```python
from build123d import *

# Parameters (mm, degrees)
SM_BASE_FLANGE_1_DEPTH  = 419.5
CUT_EXTRUDE_1_DEPTH     = 492.235686814
FILLET_1_R              = 10
HOLE_WIZARD_M12_1_D     = 10.2
HOLE_WIZARD_M12_1_DEPTH = 32.75
HOLE_WIZARD_M12_1_TIP   = 3.064389157


# Sheet-metal steps are written as plain solids
with BuildPart() as part:
    # Sketch 1 → 基体-法兰1 (new, symmetric)
    with BuildSketch(Plane(origin=(0, 0, 0), x_dir=(0, 0, -1), z_dir=(1, 0, 0))):
        with BuildLine():
            Line((-115, -111.5), (-115, -20))
            ThreePointArc((-115, -20), (-109.142135624, -5.857864376), (-95, 0))
            Line((-95, 0), (95, 0))
            ThreePointArc((95, 0), (109.142135624, -5.857864376), (115, -20))
            Line((115, -20), (115, -111.5))
            Line((115, -111.5), (105, -111.5))
            Line((105, -111.5), (105, -20))
            ThreePointArc((105, -20), (102.071067812, -12.928932188), (95, -10))
            Line((95, -10), (-95, -10))
            ThreePointArc((-95, -10), (-102.071067812, -12.928932188), (-105, -20))
            Line((-105, -20), (-105, -111.5))
            Line((-105, -111.5), (-115, -111.5))
        make_face()
    extrude(amount=SM_BASE_FLANGE_1_DEPTH, both=True)

    # Sketch 2 → 切除-拉伸1 (cut, through all)
    with BuildSketch(Plane(origin=(0, 0, -115), x_dir=(-1, 0, 0), z_dir=(0, 0, -1))):
        Polygon((-214.641016151, -111.5), (-180, -51.5), (180, -51.5), (214.641016151, -111.5), align=None)
    extrude(amount=-CUT_EXTRUDE_1_DEPTH, mode=Mode.SUBTRACT)

    # 圆角1
    fillet_1_edges = [part.edges().sort_by_distance(p)[0] for p in [
        (-214.641016151, -111.5, -110),
        (214.641016151, -111.5, -110),
        (180, -51.5, -110),
        (-180, -51.5, -110),
        (214.641016151, -111.5, 110),
        (-214.641016151, -111.5, 110),
        (-180, -51.5, 110),
        (180, -51.5, 110),
    ]]
    fillet(fillet_1_edges, radius=FILLET_1_R)

    # M12 螺纹孔1
    with Locations(Plane(origin=(0, 0, 0), x_dir=(1, 0, 0), z_dir=(0, 1, 0))):
        with Locations((-110, 50), (110, 50), (110, -50), (-110, -50)):
            Hole(HOLE_WIZARD_M12_1_D / 2, depth=HOLE_WIZARD_M12_1_DEPTH)
            with Locations((0, 0, -(HOLE_WIZARD_M12_1_DEPTH + HOLE_WIZARD_M12_1_TIP / 2))):  # 118° drill point
                Cone(0, HOLE_WIZARD_M12_1_D / 2, HOLE_WIZARD_M12_1_TIP, mode=Mode.SUBTRACT)


solid = part.part
```
Build history of the part. All positions in model axes, mm. A direction names the side the tool comes from. Give positions to 0.01 mm unless a question says otherwise; leave off trailing zeros. Loops run counter-clockwise (first coordinate to the right, second up) from the corner with the lowest first, then second, coordinate; pieces in that order, holes last.
Item 1: Slice it at D-D, the plane x = 309. List the corners of the cut face in (y, z), and give its area (3 significant figures).
Answers follow:
outline: (-111.5, -115) - (-20, -115) arc R20 ccw to (0, -95) - (0, 95) arc R20 ccw to (-20, 115) - (-111.5, 115) - (-111.5, 105) - (-20, 105) arc R10 cw to (-10, 95) - (-10, -95) arc R10 cw to (-20, -105) - (-111.5, -105) - close
area: 4,200 mm2
Item 2: Flat gauge pins, fed straight in: pin 1 (1.5 mm diameter, centred on x = -240.5, y = -18.5, fed in from -Z); pin 2 (8 mm diameter, centred on x = -41.5, z = -109, fed in from -Y); pin 3 (5 mm diameter, centred on x = -168, z = 12, fed in from -Y). Where does each tip first touch, or does it go through?
Answers follow:
pin 1: stops at z = -114.99
pin 2: stops at y = -51.5
pin 3: stops at y = -10
Item 3: Which spindle directions (+Z, -Z, +X, -X, +Y, -Y) get a long thin tool onto all of the face, cutting with end or side? Do faces 5 (the face through (6, -45, 105)), 6 (the face through (419.5, -6, -9)), 7 (the face through (-197.12, -81.15, 109.93)). Say none if no direction does.
Answers follow:
face 5: +X, -X, -Y
face 6: +Z, -Z, +X, +Y, -Y
face 7: +Z, -Z, -Y
Item 4: Slice it at C-C, the plane z = -75.5. List the corners of the cut face in (x, y), and give its area (3 significant figures).
Answers follow:
outline: (-419.5, -10) - (419.5, -10) - (419.5, 0) - (-419.5, 0) - close
area: 8,390 mm2
Item 5: Slice it at B-B, the plane x = 35.5. List the corners of the cut face in (y, z), and give its area (3 significant figures).
Answers follow:
outline: (-51.5, -115) - (-20, -115) arc R20 ccw to (0, -95) - (0, 95) arc R20 ccw to (-20, 115) - (-51.5, 115) - (-51.5, 105) - (-20, 105) arc R10 cw to (-10, 95) - (-10, -95) arc R10 cw to (-20, -105) - (-51.5, -105) - close
area: 3,000 mm2
Item 6: Pull direction Z, two halves, no side cores. Call faces 1 (the face through (6, -10, -1)), 2 (the face through (5.873, -6.014, 109.297)), 3 (the face through (6, 0, 1)), 4 (the face through (6, -45, -115)): released by +Z, released by -Z, zero draft, split by the parting line, or undercut.
Answers follow:
face 1: undercut
face 2: released by +Z
face 3: zero draft
face 4: released by -Z
Item 7: Drill centre lines: line 1 (X direction, y = -4, z = -50); line 2 (Z direction, x = 20.5, y = -27.5); line 3 (X direction, y = -7, z = 54). Where is each one in solid material? Low to high.
Answers follow:
line 1: x = -419.5 to -115.1, -104.9 to 104.9, 115.1 to 419.5
line 2: z = -115 to -105, 105 to 115
line 3: x = -419.5 to -113.16, -106.84 to 106.84, 113.16 to 419.5
Item 8: Slice it at A-A, the plane y = -29. List the corners of the cut face in (x, z), and give its area (3 significant figures).
Answers follow:
outline: (-419.5, -115) - (419.5, -115) - (419.5, -105) - (-419.5, -105) - close; (-419.5, 105) - (419.5, 105) - (419.5, 115) - (-419.5, 115) - close
area: 16,800 mm2
